Read the model definition and answer for the solid it produces. Units are mm, in the model's axes. A direction names the side the tool comes from. Coordinates: 2 decimals unless noted, no trailing zeros. Write each loop counter-clockwise with the first axis right and the second up, starting at its lowest first coordinate (ties: lowest second). Pieces come first, ordered by that corner, then holes. Notation, with made-up numbers: (43.5, -11.75) -> (81.5, -11.75) arc R26 ccw to (81.5, 26.25) -> close; hole circle Ø6 at (-29, -1). An arc over 180 degrees is marked (long way). Answer as a JSON object with one key per item and string values. Group by question number.
(1) Find section B-B (y = 0). Give the vertices of the cut face in (x, z) (3 decimals).
(2) Which of the six approach directions +Z, -Z, +X, -X, +Y, -Y give full straight-line access (tool end or side, diameter ignored) to faces 1 (the face through (6, -3, -2)), 2 (the face through (50, -3, -2)), 3 (the face through (52.39, -0.04, 0.46))?
(3) Flat-ended cylindrical pins translate along their axes: P1, Ø1.9, axis at x = 53.5, z = 0, coming from the -Y side; P2, Ø4, axis at x = 27.5, z = -3, coming from the -Y side. Find the tip coordinate at first contact, or state that the pin passes through.
(4) Find section C-C (x = 13). Give the vertices of the cut face in (y, z).
(5) Straight lines are drawn through the part: L1, parallel to X at y = 1.75, z = 0; L2, parallel to X at y = 0.5, z = -0.75; L3, parallel to Z at x = 53.5, y = 1.5. For each, find the intervals that lie inside material, in ascending order.
(6) Find section A-A (z = 0). Give the vertices of the cut face in (x, y) (3 decimals), then the cut area to 3 significant figures.
(7) For a pull along Z with two mould halves and no side action, classify faces 4 (the face through (0, 0, 0)), 5 (the face through (52.54, -0.95, 3.03)), 6 (the face through (1.355, 0.044, 0.36)) as +Z half, -Z half, draft (parallel to the pull), parting line (faces both ways), or undercut.
Autodesk Inventor part; units mm, degrees
ref_plane "Work Plane1" through (28, 0, 0) normal (-1, 0, 0) x (0, 0, 1)
ref_plane "YZ Plane" through (0, 0, 0) normal (1, 0, 0) x (0, 1, 0)
ref_plane "XZ Plane" through (0, 0, 0) normal (0, 1, 0) x (-1, 0, 0)
sketch "Sketch1" plane through (0, 0, 0) normal (0, 1, 0) x (-1, 0, 0)
  line L0 (0, 0) -> (0, 3.175)
  line L1 (0, 3.175) -> (-6, 3.175)
  line L2 (-6, 3.175) -> (-6, 4.25)
  line L3 (-6, 4.25) -> (-50, 4.25)
  line L4 (-50, 4.25) -> (-50, 3.175)
  line L5 (-50, 3.175) -> (-56, 3.175)
  line L6 (-56, 3.175) -> (-56, 0)
  line L7 (-56, 0) -> (0, 0)
  dimension "d0" = 56
  dimension "d1" = 6
  dimension "d2" = 6
  dimension "d3" = 4.25
  dimension "d4" = 3.175
revolve "Revolution1" add sketch "Sketch1" angle 360 about axis through (56, 0, 0) along (-1, 0, 0)
chamfer "Chamfer1" distance 1 angle 45 2 edges at (0, 0, -3.175) (56, 0, -3.175)
sketch "Sketch2" plane through (0, 0, 0) normal (0, 1, 0) x (-1, 0, 0)
  circle A0 centre (-2.5, 0) radius 1.2
  line L0 (0, 2.175) -> (0, -2.175)
  circle A1 centre (-53.5, 0) radius 1.2
  line L1 (-56, -2.175) -> (-56, 2.175)
  point P0 (0, 0)
  point P1 (0, 0)
  point P2 (-56, 0)
  dimension "d9" = 2.4
  dimension "d10" = 2.5
  dimension "d11" = 2.4
  dimension "d12" = 2.5
extrude "Extrusion1" cut sketch "Sketch2" along normal mid plane 10
ref_plane "Work Plane1" through (28, 0, 0) normal (-1, 0, 0) x (0, 0, 1)
properties part number "Cannon Pin" material "Iron, Cast"
Results below:
{
 "1": {"outline": "(0, -2.175) -> (1, -3.175) -> (6, -3.175) -> (6, -4.25) -> (50, -4.25) -> (50, -3.175) -> (55, -3.175) -> (56, -2.175) -> (56, 2.175) -> (55, 3.175) -> (50, 3.175) -> (50, 4.25) -> (6, 4.25) -> (6, 3.175) -> (1, 3.175) -> (0, 2.175) -> close; hole circle Ø2.4 at (2.5, 0); hole circle Ø2.4 at (53.5, 0)"},
 "2": {"face 1": "-X", "face 2": "+X", "face 3": "+Y, -Y"},
 "3": {"P1": "passes through", "P2": "stops at y = -4.13"},
 "4": {"outline": "circle Ø8.5 at (0, 0)"},
 "5": {"L1": "x = 0 to 1.3, 3.7 to 52.3, 54.7 to 56", "L2": "x = 0 to 1.56, 3.44 to 52.56, 54.44 to 56", "L3": "z = -2.8 to -1.2, 1.2 to 2.8"},
 "6": {"outline": "(0, -2.175) -> (1, -3.175) -> (1.3, -3.175) -> (1.3, 3.175) -> (1, 3.175) -> (0, 2.175) -> close; (3.7, -3.175) -> (6, -3.175) -> (6, -4.25) -> (50, -4.25) -> (50, -3.175) -> (52.3, -3.175) -> (52.3, 3.175) -> (50, 3.175) -> (50, 4.25) -> (6, 4.25) -> (6, 3.175) -> (3.7, 3.175) -> close; (54.7, -3.175) -> (55, -3.175) -> (56, -2.175) -> (56, 2.175) -> (55, 3.175) -> (54.7, 3.175) -> close", "area": "418 mm2"},
 "7": {"face 4": "draft", "face 5": "parting line", "face 6": "undercut"}
}
